from build123d import *

# Parameters (mm, degrees)
F0_W     = 28
F0_H     = 60
F1_DEPTH = 6
F2_R     = 10
F3_DEPTH = 3
F4_R     = 5.5
F4_R_2   = 1.25
F5_DEPTH = 3.001
F7_SIZE  = 7


# Not quite as in the source:
# - a fillet or chamfer that OpenCascade refuses, or shapes differently, is made with other operations: its cross-section is extruded or revolved along the edge and cut away or added


with BuildPart() as f1:
    # F0 (on Top) → F1 (new body)
    with BuildSketch(Plane.XY):
        with Locations((0, 16)):
            Rectangle(F0_W, F0_H)
    extrude(amount=F1_DEPTH)

    # F2 (on face) → F3 (cut)
    with BuildSketch(Plane.XY.offset(6)):
        Circle(F2_R)
    extrude(amount=-F3_DEPTH, mode=Mode.SUBTRACT)

    # F4 (on face) → F5 (cut, through all)
    with BuildSketch(Plane.XY.offset(3)):
        Circle(F4_R)
        with Locations((0, 7.0710678119)):
            Circle(F4_R_2)
        with Locations((7.0710678119, 0)):
            Circle(F4_R_2)
        with Locations((0, -7.0710678119)):
            Circle(F4_R_2)
        with Locations((-7.0710678119, 0)):
            Circle(F4_R_2)
    extrude(amount=-F5_DEPTH, mode=Mode.SUBTRACT)

    # F6: chamfer of 1 on 1 edges, made by hand

    # F6_s1 → F6_t2 (revolve, cut)
    with BuildSketch(Plane.XZ):
        Polygon((6.5, 0), (5.5, 1), (5.5, 0), align=None)
    revolve(axis=Axis((0, 0, 0), (0, 0, 1)), mode=Mode.SUBTRACT)

    # F7
    f7_edges = [f1.edges().sort_by_distance(p)[0] for p in [
        (14, -14, 3),
        (-14, -14, 3),
        (14, 46, 3),
        (-14, 46, 3),
    ]]
    chamfer(f7_edges, length=F7_SIZE)


solid = f1.part
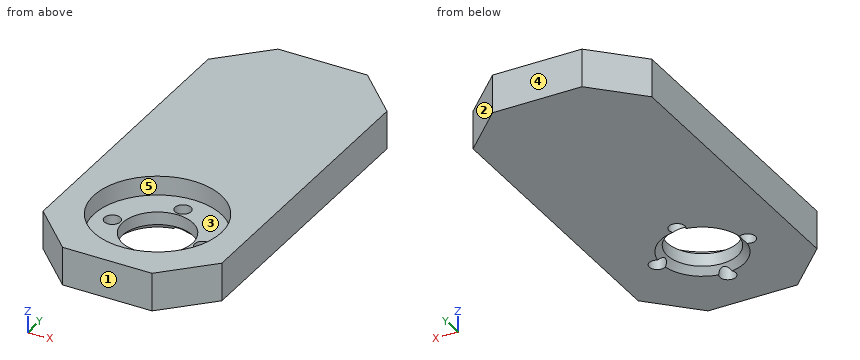
Verification items for the finished model (mm, model axes). Face numbers are marked on the shaded views. A direction names the side the tool comes from. Give positions to 0.01 mm unless a question says otherwise; leave off trailing zeros. Write each loop counter-clockwise with the first axis right and the second up, starting at its lowest first coordinate (ties: lowest second). Pieces come first, ordered by that corner, then holes.
(1) Material ranges on line 1 (Y direction, x = 0, z = 1.05); line 2 (Z direction, x = -8.25, y = -2.5); line 3 (Y direction, x = 0, z = 3.75), recorded low to high.
(2) Cross-section at D-D (z = 1.75). Enter the section's corners in (x, y).
(3) Gauge pin test, flat ends, axial feed: pin 1 (4 mm diameter, centred on x = 0, y = -7.07, fed in from +Z); pin 2 (1.5 mm diameter, centred on x = 10, z = 2, fed in from +Y); pin 3 (3 mm diameter, centred on x = -9, z = 2.5, fed in from -Y). Record the tip position at first contact, or that the pin passes through.
(4) Cross-section at C-C (y = 0). Enter the section's corners in (x, z).
(5) Cross-section at B-B (x = 0). Enter the section's corners in (y, z).
(6) Cross-section at A-A (z = 4.25). Enter the section's corners in (x, y), plus the area to 3 significant figures.
(7) Mould release check, pull along Y, two halves, no side actions. Record for the marked faces 1, 2 and 3: +Y half, -Y half, draft (parallel to the pull), parting line (faces both ways), or undercut.
(8) Access from +Z, -Z, +X, -X, +Y, -Y to the whole of each face (thin tool, end or side, straight path). Record for the marked faces 4 and 5.
Worked out:
1. line 1: y = -14 to -8.32, -5.82 to -5.5, 5.5 to 5.82, 8.32 to 46
1. line 2: z = 0 to 3
1. line 3: y = -14 to -10, 10 to 46
2. outline: (-14, -7) - (-7, -14) - (7, -14) - (14, -7) - (14, 39) - (7, 46) - (-7, 46) - (-14, 39) - close; hole circle Ø2.5 at (-7.07, 0); hole circle Ø11 at (0, 0); hole circle Ø2.5 at (0, -7.07); hole circle Ø2.5 at (0, 7.07); hole circle Ø2.5 at (7.07, 0)
3. pin 1: stops at z = 3
3. pin 2: stops at y = 43.75
3. pin 3: stops at y = -13.5
4. outline: (-14, 0) - (-8.32, 0) - (-8.32, 3) - (-10, 3) - (-10, 6) - (-14, 6) - close; (-5.82, 0.68) - (-5.5, 1) - (-5.5, 3) - (-5.82, 3) - close; (5.5, 1) - (5.82, 0.68) - (5.82, 3) - (5.5, 3) - close; (8.32, 0) - (14, 0) - (14, 6) - (10, 6) - (10, 3) - (8.32, 3) - close
5. outline: (-14, 0) - (-8.32, 0) - (-8.32, 3) - (-10, 3) - (-10, 6) - (-14, 6) - close; (-5.82, 0.68) - (-5.5, 1) - (-5.5, 3) - (-5.82, 3) - close; (5.5, 1) - (5.82, 0.68) - (5.82, 3) - (5.5, 3) - close; (8.32, 0) - (46, 0) - (46, 6) - (10, 6) - (10, 3) - (8.32, 3) - close
6. outline: (-14, -7) - (-7, -14) - (7, -14) - (14, -7) - (14, 39) - (7, 46) - (-7, 46) - (-14, 39) - close; hole circle Ø20 at (0, 0)
6. area: 1,270 mm2
7. face 1: -Y half
7. face 2: +Y half
7. face 3: undercut
8. face 4: +Z, -Z, +X, -X, +Y
8. face 5: +Z
